Could you check a few things on this model? Use its own coordinates, in mm. Face numbers are marked on the shaded views. A direction names the side the tool comes from. Give positions to 0.01 mm unless a question says otherwise; leave off trailing zeros. Write each loop counter-clockwise with the first axis right and the second up, starting at its lowest first coordinate (ties: lowest second). Pieces come first, ordered by that corner, then holes. Notation, with made-up numbers: (29, 39.5) - (46, 39.5) arc R17 cw to (46, 64.5) - close; hole circle Ø11 at (51, -9). An arc over 180 degrees is marked (long way). Answer in a Markdown table with one row per item.
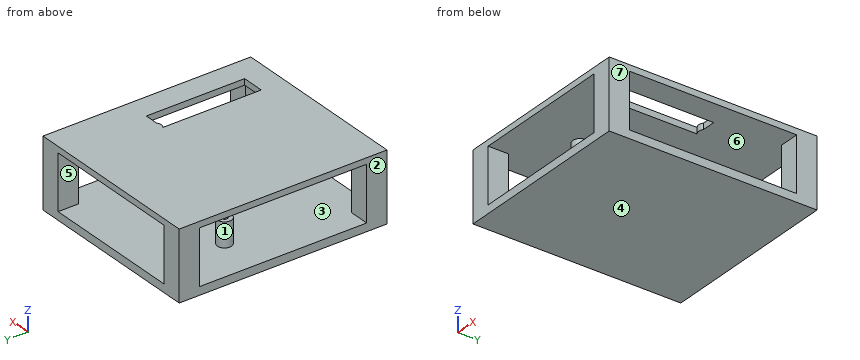
Autodesk Fusion 360 part; units mm, degrees
sketch "Esquisse1" plane through (0, 0, 0) normal (0, 0, 1) x (1, 0, 0)
  line L0 (0, 0) -> (70, 0)
  line L1 (70, 0) -> (70, 82.5)
  line L2 (70, 82.5) -> (0, 82.5)
  line L3 (0, 82.5) -> (0, 0)
  circle A0 centre (43.89, 2.5) radius 1.5
  circle A1 centre (10.87, 54.57) radius 1.5
  circle A2 centre (59.13, 53.3) radius 1.5
  line L4 (-10, -10) -> (80, -10)
  line L5 (80, -10) -> (80, 92.5)
  line L6 (80, 92.5) -> (-10, 92.5)
  line L7 (-10, 92.5) -> (-10, -10)
  line L8 (80, 92.5) -> (70, 92.5)
  line L9 (70, 92.5) -> (70, 82.5)
  line L10 (70, 82.5) -> (80, 82.5)
  line L11 (80, 82.5) -> (80, 92.5)
  line L12 (80, -10) -> (70, -10)
  line L13 (70, -10) -> (70, 0)
  line L14 (70, 0) -> (80, 0)
  line L15 (80, 0) -> (80, -10)
  line L16 (0, 0) -> (-10, 0)
  line L17 (-10, 0) -> (-10, -10)
  line L18 (-10, -10) -> (0, -10)
  line L19 (0, -10) -> (0, 0)
  line L20 (0, 82.5) -> (-10, 82.5)
  line L21 (-10, 82.5) -> (-10, 92.5)
  line L22 (-10, 92.5) -> (0, 92.5)
  line L23 (0, 92.5) -> (0, 82.5)
  line L24 (68, 2) -> (57, 2)
  line L25 (57, 2) -> (57, 50.5)
  line L26 (57, 50.5) -> (68, 50.5)
  line L27 (68, 50.5) -> (68, 2)
  line L28 (2, 50.5) -> (13, 50.5)
  line L29 (13, 50.5) -> (13, 2)
  line L30 (13, 2) -> (2, 2)
  line L31 (2, 2) -> (2, 50.5)
  line L32 (68, 80) -> (65.5, 80)
  line L33 (65.5, 80) -> (65.5, 75)
  line L34 (65.5, 75) -> (68, 75)
  line L35 (68, 75) -> (68, 80)
  line L36 (2, 80) -> (4.5, 80)
  line L37 (4.5, 80) -> (4.5, 75)
  line L38 (4.5, 75) -> (2, 75)
  line L39 (2, 75) -> (2, 80)
  circle A3 centre (10.87, 54.57) radius 3.5
  circle A4 centre (59.13, 53.3) radius 3.5
  circle A5 centre (43.89, 2.5) radius 3.5
  dimension "d1" = 70
  dimension "d2" = 82.5
  dimension "d3" = 3
  dimension "d4" = 26.11
  dimension "d5" = 2.5
  dimension "d6" = 3
  dimension "d7" = 10.87
  dimension "d8" = 27.93
  dimension "d9" = 3
  dimension "d10" = 29.2
  dimension "d12" = 90
  dimension "d13" = 102.5
  dimension "d14" = 10
  dimension "d15" = 10
  dimension "d16" = 10.87
  dimension "d17" = 11
  dimension "d18" = 48.5
  dimension "d19" = 2
  dimension "d20" = 2
  dimension "d21" = 11
  dimension "d22" = 48.5
  dimension "d23" = 2
  dimension "d24" = 2
  dimension "d25" = 2.5
  dimension "d26" = 5
  dimension "d27" = 2.5
  dimension "d28" = 5
  dimension "d29" = 2
  dimension "d30" = 2.5
  dimension "d31" = 2
  dimension "d32" = 2.5
  dimension "d35" = 7
  dimension "d36" = 7
  dimension "d37" = 7
extrude "Extrusion1" add sketch "Esquisse1" against normal blind 4 contours L0 L1 L2 L3 A5 | L3 L7 L16 L20 | L4 L7 L16 L17 L18 L19 | L0 L4 L13 L19 A5 | L0 A5 | L0 A5 | L2 L6 L9 L23 | L6 L7 L20 L21 L22 L23 | L1 L5 L10 L14 | L5 L6 L8 L9 L10 L11 | L4 L5 L12 L13 L14 L15 | A0 | A1 | A2 | L24 L25 L26 L27 A4 | L26 A4 | L26 A4 | L28 L29 L30 L31 | L32 L33 L34 L35 | L36 L37 L38 L39 | A3
extrude "Extrusion2" add sketch "Esquisse1" along normal blind 12 contours L0 A5 | L0 A5 | L26 A4 | L26 A4 | A3
extrude "Extrusion3" add sketch "Esquisse1" along normal blind 27 contours L4 L7 L16 L17 L18 L19 | L6 L7 L20 L21 L22 L23 | L5 L6 L8 L9 L10 L11 | L4 L5 L12 L13 L14 L15
sketch "Esquisse3" plane through (0, 0, 27) normal (0, 0, 1) x (-1, 0, 0)
  line L0 (-80, 0) -> (-70, 0)
  line L1 (-70, 0) -> (-70, 10)
  line L2 (-70, 10) -> (-80, 10)
  line L3 (-80, 10) -> (-80, 0)
  line L4 (10, 10) -> (-80, 10)
  line L5 (-80, 10) -> (-80, -92.5)
  line L6 (-80, -92.5) -> (10, -92.5)
  line L7 (10, -92.5) -> (10, 10)
  dimension "d42" = 90
  dimension "d43" = 102.5
extrude "Extrusion4" add sketch "Esquisse3" along normal blind 3
extrude "Extrusion5" cut sketch "Esquisse1" along normal blind 40 contours L24 L25 L26 L27 A4
1) Will these pins go through, and if not, where does the flat tip stop? P1, Ø10, axis at x = 52.5, z = 15, coming from the +Y side; P2, Ø6, axis at y = 78, z = 12, coming from the -X side.
Check values:
| item | result |
|---|---|
| P1 | stops at y = 55.61 |
| P2 | passes through |
2) Imagine slicing it at A-A (x = 43.89). List the corners of the cut face in (y, z) for me.
Check values:
| item | result |
|---|---|
| outline | (-10, -4) - (92.5, -4) - (92.5, 0) - (6, 0) - (6, 12) - (4, 12) - (4, 0) - (1, 0) - (1, 12) - (-1, 12) - (-1, 0) - (-10, 0) - close; (-10, 27) - (92.5, 27) - (92.5, 30) - (-10, 30) - close |
3) On a 3-axis mill with a long thin cutter (end or side, diameter ignored), from which of +Z, -Z, +X, -X, +Y, -Y can I reach the whole of each face in a straight line? I mean the marked faces 5, 6 and 7. Say none if no direction works.
Check values:
| item | result |
|---|---|
| face 5 | +Y, -Y |
| face 6 | none |
| face 7 | +Z, -Z, +X, +Y, -Y |
4) We'd pull the mould along Z, two halves only. Please class the marked faces 1, 2, 3 and 4: +Z half, -Z half, draft (parallel to the pull), parting line (faces both ways), or undercut.
Check values:
| item | result |
|---|---|
| face 1 | undercut |
| face 2 | draft |
| face 3 | undercut |
| face 4 | -Z half |
5) Imagine slicing it at C-C (x = 59.13). List the corners of the cut face in (y, z) for me, then the cut area to 3 significant figures.
Check values:
| item | result |
|---|---|
| outline | (-10, -4) - (92.5, -4) - (92.5, 0) - (56.8, 0) - (56.8, 12) - (54.8, 12) - (54.8, 0) - (51.8, 0) - (51.8, 12) - (49.8, 12) - (49.8, 0) - (-10, 0) - close; (-10, 27) - (2, 27) - (2, 30) - (-10, 30) - close; (49.8, 27) - (92.5, 27) - (92.5, 30) - (49.8, 30) - close |
| area | 622 mm2 |
6) Imagine slicing it at B-B (z = 16). List the corners of the cut face in (x, y) for me, then the cut area to 3 significant figures.
Check values:
| item | result |
|---|---|
| outline | (-10, -10) - (0, -10) - (0, 0) - (-10, 0) - close; (-10, 82.5) - (0, 82.5) - (0, 92.5) - (-10, 92.5) - close; (70, -10) - (80, -10) - (80, 0) - (70, 0) - close; (70, 82.5) - (80, 82.5) - (80, 92.5) - (70, 92.5) - close |
| area | 400 mm2 |
7) Imagine slicing it at D-D (y = 80.5). List the corners of the cut face in (x, z) for me, then the cut area to 3 significant figures.
Check values:
| item | result |
|---|---|
| outline | (-10, -4) - (80, -4) - (80, 0) - (-10, 0) - close; (-10, 27) - (80, 27) - (80, 30) - (-10, 30) - close |
| area | 630 mm2 |
8) If I drill on line 1 (Y direction, x = 43.89, z = 5.75); line 2 (Y direction, x = 59.13, z = 9); line 3 (X direction, y = 83.5, z = 13), over which ranges is the centre line in solid material (lowest first)?
Check values:
| item | result |
|---|---|
| line 1 | y = -1 to 1, 4 to 6 |
| line 2 | y = 49.8 to 51.8, 54.8 to 56.8 |
| line 3 | x = -10 to 0, 70 to 80 |
